Design review of the part built by this model. Coordinates are the model's own, in mm. Face numbers are marked on the shaded views. A direction names the side the tool comes from. Round coordinates to 2 decimals unless told otherwise and drop trailing zeros. Order: outer loops, then holes, each group sorted by start corner. A loop starts at its lowest first (then second) coordinate and runs counter-clockwise, first axis right, second up. Notation, with made-up numbers: (6.25, 45.5) - (36.25, 45.5) arc R9 ccw to (36.25, 50.5) - close; hole circle Ø3 at (69.25, 23.5). An arc over 180 degrees is marked (long way). Write item = value, one per line.
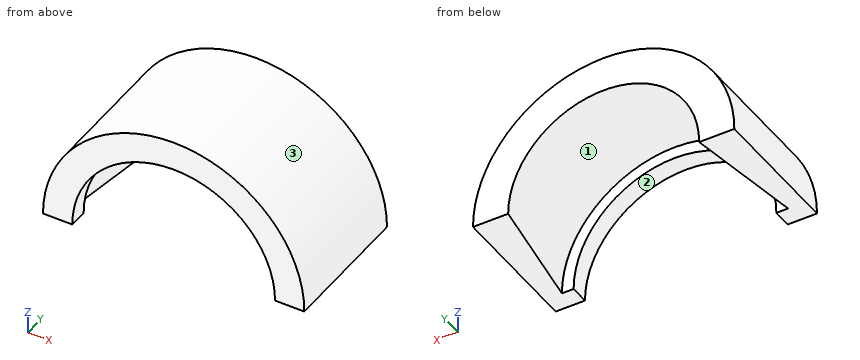
from build123d import *

# Parameters (mm, degrees)
REVOLUTION_ANGLE = -180


with BuildPart() as part:
    # Sketch → Revolution (revolve)
    with BuildSketch(Plane.XY):
        Polygon((17.3, 0), (17.3, 3.2), (19.3, 3.2), (16.3, 23.3), (22.3, 23.3), (22.3, 0), align=None)
    revolve(axis=Axis((0, 0, 0), (0, 1, 0)), revolution_arc=REVOLUTION_ANGLE)


solid = part.part
Item 1: For line 1 along X through (y, z) = (9.25, 5); line 2 along X through (y, z) = (7.5, 8); line 3 along Z through (x, y) = (11, 6), list the stretches that pass through material, from the lowest coordinate up. Write a range as [from, to].
Data:
line_1 = [-21.73, -17.7], [17.7, 21.73]
line_2 = [-20.82, -16.86], [16.86, 20.82]
line_3 = [15.35, 19.4]
Item 2: Insertion check: P1, Ø2, axis at y = 5, z = 15.5, coming from the +X side; P2, Ø2, axis at x = -8.5, y = 2.5, coming from the +Z side; P3, Ø2, axis at y = 12, z = 15, coming from the -X side. Each pin has a flat end and moves straight along its axis. Give the tip position at first contact, or say it passes through.
Data:
P1 = 16.94
P2 = 21
P3 = -17.36
Item 3: Take a section at B-B, the plane y = 17.25. State the section outline as (x, z) points.
Data:
outline = (-22.3, 0) - (-17.2, 0) arc R17.2 cw to (17.2, 0) - (22.3, 0) arc R22.3 ccw to start
Item 4: For the marked faces 1, 2 and 3, list the 3-axis set-ups (+Z, -Z, +X, -X, +Y, -Y) from which the entire face can be reached by the end or side of a thin tool; tool diameter is ignored.
Data:
face_1 = -Z
face_2 = -Z, -Y
face_3 = +Z, +Y, -Y
Item 5: Take a section at C-C, the plane y = 21. State the section outline as (x, z) points.
Data:
outline = (-22.3, 0) - (-16.64, 0) arc R16.64 cw to (16.64, 0) - (22.3, 0) arc R22.3 ccw to start
Item 6: Take a section at A-A, the plane x = 0. State the section outline as (y, z) points, and give its area (3 significant figures).
Data:
outline = (0, 17.3) - (3.2, 17.3) - (3.2, 19.3) - (23.3, 16.3) - (23.3, 22.3) - (0, 22.3) - close
area = 106 mm2
